from build123d import *

# Parameters (mm, degrees)
BOSS_EXTRUDE1_DEPTH = 388
SKETCH2_R           = 1.25
CUT_EXTRUDE1_DEPTH  = 202


with BuildPart() as part:
    # Sketch1 → Boss-Extrude1 (new body)
    with BuildSketch(Plane(origin=(0, 0, 0), x_dir=(1, 0, 0), z_dir=(0, 1, 0))):
        with BuildLine():
            Line((0, 85), (0, 83))
            ThreePointArc((0, 83), (83, 0), (0, -83))
            Line((0, -83), (0, -85))
            ThreePointArc((0, -85), (85, 0), (0, 85))
        make_face()
    extrude(amount=BOSS_EXTRUDE1_DEPTH)

    # Sketch2 → Cut-Extrude1 (cut)
    with BuildSketch(Plane(origin=(0, 0, 0), x_dir=(0, 0, -1), z_dir=(1, 0, 0))):
        with Locations(Location((0, 385, 0), (0, 0, 180))):
            Circle(SKETCH2_R)
        with Locations(Location((0, 3, 0), (0, 0, 180))):
            Circle(SKETCH2_R)
    extrude(amount=CUT_EXTRUDE1_DEPTH, mode=Mode.SUBTRACT)


solid = part.part
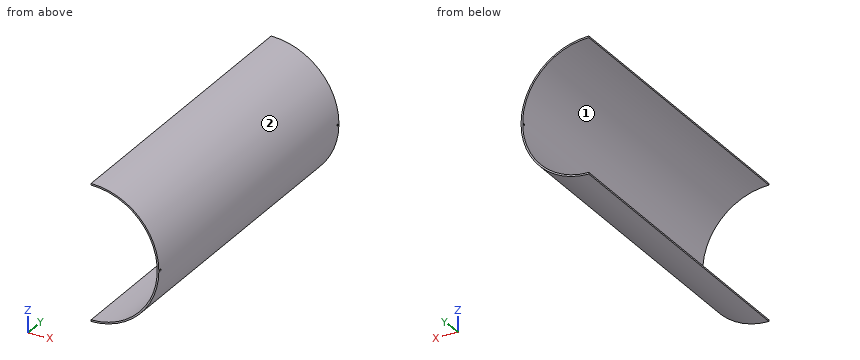
CAD build for the part. Positions are in the model's coordinates, mm. Face numbers are marked on the shaded views. Give positions to 0.01 mm unless a question says otherwise; leave off trailing zeros. Write each loop counter-clockwise with the first axis right and the second up, starting at its lowest first coordinate (ties: lowest second). Pieces come first, ordered by that corner, then holes. Notation, with made-up numbers: (21, -33.5) -> (40, -33.5) arc R22 cw to (40, 1.5) -> close; hole circle Ø3 at (-15, 66.5). An arc over 180 degrees is marked (long way). Return JSON: item names as keys, results as strings.
Item 1: Band-saw the part on C-C (x = 37.5). List the corners of the cut face in (y, z).
Answer below:
{"outline": "(0, -76.28) -> (388, -76.28) -> (388, -74.05) -> (0, -74.05) -> close; (0, 74.05) -> (388, 74.05) -> (388, 76.28) -> (0, 76.28) -> close"}
Item 2: Band-saw the part on D-D (z = 11). List the corners of the cut face in (x, y).
Answer below:
{"outline": "(82.27, 0) -> (84.29, 0) -> (84.29, 388) -> (82.27, 388) -> close"}
Item 3: Two-plate mould, pull along Z, no slides. Class the marked faces 1 and 2: +Z half, -Z half, draft (parallel to the pull), parting line (faces both ways), or undercut.
Answer below:
{"face 1": "undercut", "face 2": "parting line"}
Item 4: Band-saw the part on A-A (x = 73). List the corners of the cut face in (y, z), then the cut area to 3 significant figures.
Answer below:
{"outline": "(0, -43.54) -> (388, -43.54) -> (388, -39.5) -> (0, -39.5) -> close; (0, 39.5) -> (388, 39.5) -> (388, 43.54) -> (0, 43.54) -> close", "area": "3,140 mm2"}
Item 5: Drill centre lines: probe 1 along Y at (x, z) = (84, 0); probe 2 along Z at (x, y) = (22, 205); probe 3 along Z at (x, y) = (74, 152.5). Where is each one in solid material? Low to high.
Answer below:
{"probe 1": "y = 0 to 1.75, 4.25 to 383.75, 386.25 to 388", "probe 2": "z = -82.1 to -80.03, 80.03 to 82.1", "probe 3": "z = -41.82 to -37.59, 37.59 to 41.82"}
Item 6: Drop flat-ended pins along their axis: pin 1 (4 mm diameter, centred on y = 193.5, z = 49.5, fed in from +X); pin 2 (6 mm diameter, centred on x = 46, y = 68.5, fed in from +Z); pin 3 (6 mm diameter, centred on y = 82.5, z = -67.5, fed in from -X). Give the stop position or say it passes through.
Answer below:
{"pin 1": "stops at x = 70.49", "pin 2": "stops at z = 73.32", "pin 3": "stops at x = 43.8"}
Item 7: Band-saw the part on B-B (y = 304). List the corners of the cut face in (x, z), then the cut area to 3 significant figures.
Answer below:
{"outline": "(0, -85) arc R85 ccw to (0, 85) -> (0, 83) arc R83 cw to (0, -83) -> close", "area": "528 mm2"}
